Part model, mm, in its own coordinate system. Give positions to 0.01 mm unless a question says otherwise; leave off trailing zeros. Write each loop counter-clockwise with the first axis right and the second up, starting at its lowest first coordinate (ties: lowest second). Pieces come first, ordered by that corner, then holes. Notation, with made-up numbers: M 17,-13 L 74,-13 A13 ccw 74,-6 Z; hole C 2.25,27.5 d1. An arc over 180 degrees is marked long. Use CSV: the item, a comma, the result in double quotes. Start each with the question number.
Item 1: Cut at B-B (x = 2.25). List the corners of the cut face in (y, z), then the cut area to 3 significant figures.
Item 2: Cut at A-A (y = -3). List the corners of the cut face in (x, z).
Item 3: Cut at D-D (z = -11.25). List the corners of the cut face in (x, y).
Item 4: Drill centre lines: line 1 (Y direction, x = 7.25, z = -4.75); line 2 (Z direction, x = 5.25, y = 0); line 3 (Z direction, x = 8.5, y = -11.5). Where is each one in solid material? Low to high. Write a range as [from, to].
Item 5: Pin check, flat tips, straight feed: pin 1 (5 mm diameter, centred on x = 8.5, z = -11.5, fed in from +Y); pin 2 (4 mm diameter, centred on x = 3.5, z = -8, fed in from -Y). Stop position of each tip, or through.
Item 6: Cut at C-C (z = -2). List the corners of the cut face in (x, y), then the cut area to 3 significant figures.
from build123d import *

# Parameters (mm, degrees)
PAD_DEPTH = 10


with BuildPart() as part:
    # Sketch → Pad (new body)
    with BuildSketch(Plane.YZ):
        with BuildLine():
            ThreePointArc((-1, 0), (0, -9.898979), (1, 0))
            Line((1, 0), (16, 0))
            Line((16, 0), (16, -3))
            Line((16, -3), (7.77135, -3))
            ThreePointArc((-7.77135, -3), (0, -12.898979), (7.77135, -3))
            Line((-16, -3), (-7.77135, -3))
            Line((-16, 0), (-16, -3))
            Line((-1, 0), (-16, 0))
        make_face()
    extrude(amount=PAD_DEPTH)


solid = part.part
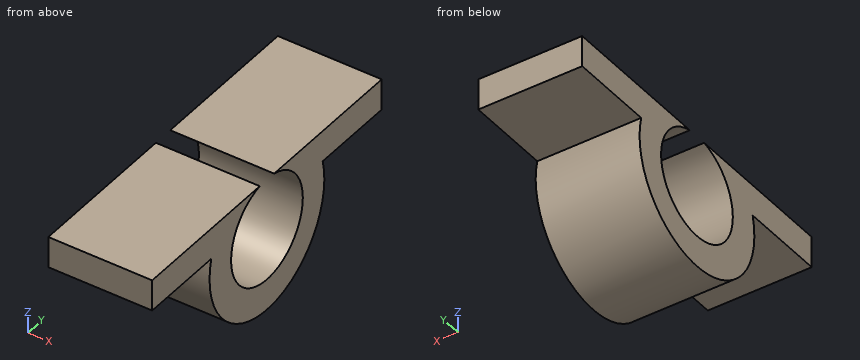
Worked answers:
1,outline,"M -16,-3 L -7.77,-3 A8 ccw long 7.77,-3 L 16,-3 L 16,0 L 1,0 A5 cw long -1,0 L -16,0 Z"
1,area,"148 mm^2"
2,outline,"M 0,-12.32 L 10,-12.32 L 10,-8.9 L 0,-8.9 Z; M 0,-0.9 L 10,-0.9 L 10,0 L 0,0 Z"
3,outline,"M 0,-4.86 L 10,-4.86 L 10,4.86 L 0,4.86 Z"
4,line 1,"y = [-8, -5], [5, 8]"
4,line 2,"z = [-12.9, -9.9]"
4,line 3,"z = [-3, 0]"
5,pin 1,"stops at y = 6.87"
5,pin 2,"stops at y = -7.92"
6,outline,"M 0,-16 L 10,-16 L 10,-4.07 L 0,-4.07 Z; M 0,4.07 L 10,4.07 L 10,16 L 0,16 Z"
6,area,"239 mm^2"
